```python
from build123d import *

# Parameters (mm, degrees)
F0_R     = 75.5
F0_R_2   = 67.5
F1_DEPTH = 10
F3_DEPTH = 6
F4_DEPTH = 5


with BuildPart() as f1:
    # F0 (on Top) → F1 (new body)
    with BuildSketch(Plane.XY):
        Circle(F0_R)
        Circle(F0_R_2, mode=Mode.SUBTRACT)
    extrude(amount=F1_DEPTH)

    # F2 (on face) → F3 (cut)
    with BuildSketch(Plane.XY.offset(10)):
        with BuildLine():
            Line((1.25, 71.4890725916), (1.25, 74.5))
            Line((1.25, 74.5), (-1.25, 74.5))
            Line((-1.25, 74.5), (-1.25, 71.4890725916))
            ThreePointArc((-1.25, 71.4890725916), (0, 71.5), (1.25, 71.4890725916))
        make_face()
        with BuildLine():
            Line((1.25, 67.4884249335), (1.25, 71.4890725916))
            ThreePointArc((1.25, 71.4890725916), (0, 71.5), (-1.25, 71.4890725916))
            Line((-1.25, 71.4890725916), (-1.25, 67.4884249335))
            ThreePointArc((-1.25, 67.4884249335), (0, 67.5), (1.25, 67.4884249335))
        make_face()
        with BuildLine():
            Line((-1.25, -67.4884249335), (-1.25, -71.4890725916))
            ThreePointArc((-1.25, -71.4890725916), (0, -71.5), (1.25, -71.4890725916))
            Line((1.25, -71.4890725916), (1.25, -67.4884249335))
            ThreePointArc((1.25, -67.4884249335), (0, -67.5), (-1.25, -67.4884249335))
        make_face()
        with BuildLine():
            ThreePointArc((1.25, -71.4890725916), (0, -71.5), (-1.25, -71.4890725916))
            Line((-1.25, -71.4890725916), (-1.25, -74.5))
            Line((-1.25, -74.5), (1.25, -74.5))
            Line((1.25, -74.5), (1.25, -71.4890725916))
        make_face()
    extrude(amount=-F3_DEPTH, mode=Mode.SUBTRACT)

    # F2 (on face) → F4 (cut)
    with BuildSketch(Plane.XY.offset(10)):
        with BuildLine():
            ThreePointArc((71.5, 0), (50.9981617316, 50.114244482), (1.25, 71.4890725916))
            Line((1.25, 71.4890725916), (1.25, 67.4884249335))
            ThreePointArc((1.25, 67.4884249335), (48.16962217, 47.2857007984), (67.5, 0))
            ThreePointArc((67.5, 0), (48.16962217, -47.2857007984), (1.25, -67.4884249335))
            Line((1.25, -67.4884249335), (1.25, -71.4890725916))
            ThreePointArc((1.25, -71.4890725916), (50.9981617316, -50.114244482), (71.5, 0))
        make_face()
        with BuildLine():
            Line((-1.25, 67.4884249335), (-1.25, 71.4890725916))
            ThreePointArc((-1.25, 71.4890725916), (-71.5, 0), (-1.25, -71.4890725916))
            Line((-1.25, -71.4890725916), (-1.25, -67.4884249335))
            ThreePointArc((-1.25, -67.4884249335), (-67.5, 0), (-1.25, 67.4884249335))
        make_face()
    extrude(amount=-F4_DEPTH, mode=Mode.SUBTRACT)


solid = f1.part
```
Read the model definition and answer for the solid it produces. Units are mm, in the model's axes. A direction names the side the tool comes from. Coordinates: 2 decimals unless noted, no trailing zeros. Loops run counter-clockwise (first coordinate to the right, second up) from the corner with the lowest first, then second, coordinate; pieces in that order, holes last. Notation, with made-up numbers: (29, 11.25) -> (79, 11.25) arc R36 ccw to (79, 48.25) -> close; hole circle Ø9 at (51.25, 69.5). An arc over 180 degrees is marked (long way). Return JSON: item names as keys, results as strings.
Item 1: Find section C-C (z = 2). Determine the outline of the cut face in (x, y).
Answers:
{"outline": "circle Ø151 at (0, 0); hole circle Ø135 at (0, 0)"}
Item 2: For a pull along X with two mould halves and no side action, classify faces 1 (the flat face through (-1.25, -73, 7)), 2 (the cylindrical face through (72.014, 22.678, 4.93)), 3 (the flat face through (-45, -56, 10)) as +X half, -X half, draft (parallel to the pull), parting line (faces both ways), or undercut.
Answers:
{"face 1": "undercut", "face 2": "parting line", "face 3": "draft"}
Item 3: Flat-ended cylindrical pins translate along their axes: P1, Ø1, axis at x = -20.5, z = 5, coming from the +Y side; P2, Ø0.8, axis at x = 0.5, y = -70.5, coming from the +Z side; P3, Ø3, axis at x = 0.5, z = 6, coming from the -Y side. Find the tip coordinate at first contact, or state that the pin passes through.
Answers:
{"P1": "stops at y = 72.8", "P2": "stops at z = 4", "P3": "stops at y = -75.5"}
Item 4: Find the intervals of material crossed by probe 1 along X at (y, z) = (-1, 7); probe 2 along Y at (x, z) = (0, 1.9); probe 3 along Y at (x, z) = (-39.5, 2), in increasing order.
Answers:
{"probe 1": "x = -75.49 to -71.49, 71.49 to 75.49", "probe 2": "y = -75.5 to -67.5, 67.5 to 75.5", "probe 3": "y = -64.34 to -54.74, 54.74 to 64.34"}
Item 5: Find section A-A (y = 0). Determine the outline of the cut face in (x, z).
Answers:
{"outline": "(-75.5, 0) -> (-67.5, 0) -> (-67.5, 5) -> (-71.5, 5) -> (-71.5, 10) -> (-75.5, 10) -> close; (67.5, 0) -> (75.5, 0) -> (75.5, 10) -> (71.5, 10) -> (71.5, 5) -> (67.5, 5) -> close"}
Item 6: Find section B-B (x = 47). Determine the outline of the cut face in (y, z), plus the area to 3 significant figures.
Answers:
{"outline": "(-59.09, 0) -> (-48.45, 0) -> (-48.45, 5) -> (-53.88, 5) -> (-53.88, 10) -> (-59.09, 10) -> close; (48.45, 0) -> (59.09, 0) -> (59.09, 10) -> (53.88, 10) -> (53.88, 5) -> (48.45, 5) -> close", "area": "158 mm2"}
Item 7: For faces 4 (the cylindrical face through (-53.57, -41.07, 2.46)), 5 (the cylindrical face through (-71.483, 1.555, 7.535)), determine the directions among +Z, -Z, +X, -X, +Y, -Y from which every point of the face is accessible in a straight line to the end or side of a thin tool.
Answers:
{"face 4": "+Z, -Z", "face 5": "+Z"}
